Could you check a few things on this drawing? It's one solid part, dimensions in mm from its lowest x, y, z. A direction names the side the tool comes from. Round coordinates to 2 decimals unless told otherwise and drop trailing zeros. Loops run counter-clockwise (first coordinate to the right, second up) from the corner with the lowest first, then second, coordinate; pieces in that order, holes last. Notation, with made-up numbers: (-4, 83) -> (38, 83) arc R14 ccw to (38, 95) -> close; hole circle Ø5 at (53, 79.25). An arc over 180 degrees is marked (long way). Write each question's results on one line, items separated by ' | '.
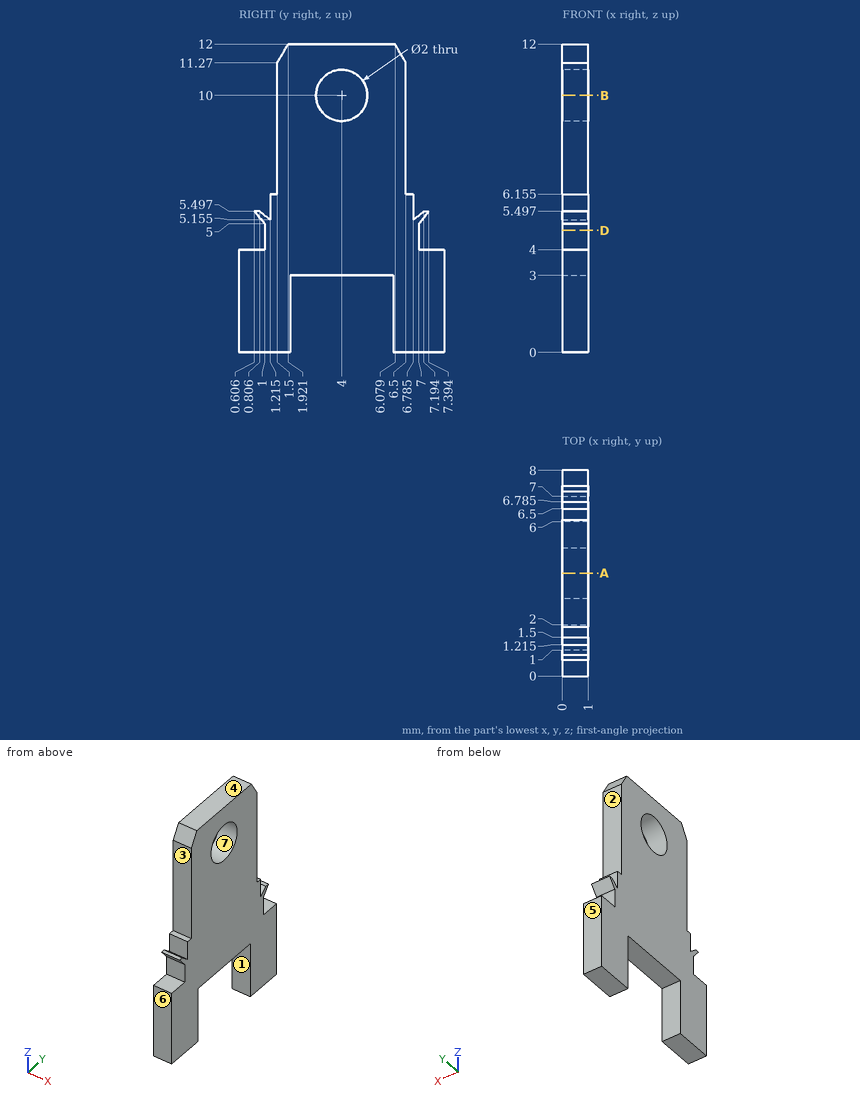
1) I want a section at B-B, the plane z = 10. Write out the boundary of the cut face in (x, y).
Model answer:
outline: (0, 1.5) -> (1, 1.5) -> (1, 3) -> (0, 3) -> close; (0, 5) -> (1, 5) -> (1, 6.5) -> (0, 6.5) -> close
2) For the marked faces 1, 2, 3 and 4, which set-ups out of +Z, -Z, +X, -X, +Y, -Y let a thin tool reach every point of the face, with its end or its side?
Model answer:
face 1: -Z, +X, -X | face 2: +Z, +X, -X, +Y | face 3: +Z, +X, -X, -Y | face 4: +Z, +X, -X, +Y, -Y
3) If we mould it in two halves opening along Y, with no side actions, what happens to the marked faces 5, 6 and 7? For each: released by +Y, released by -Y, zero draft, split by the parting line, or undercut.
Model answer:
face 5: released by +Y | face 6: released by -Y | face 7: undercut
4) I need wall thicknesses on line 1 (Z direction, x = 0.35, y = 4); line 2 (Y direction, x = 0.65, z = 10); line 3 (Y direction, x = 0.95, z = 2). Which ranges of each line are inside material? Lowest first, please.
Model answer:
line 1: z = 3 to 9, 11 to 12 | line 2: y = 1.5 to 3, 5 to 6.5 | line 3: y = 0 to 2, 6 to 8
5) I want a section at D-D, the plane z = 4.75. Write out the boundary of the cut face in (x, y).
Model answer:
outline: (0, 1) -> (1, 1) -> (1, 7) -> (0, 7) -> close
6) I want a section at A-A, the plane y = 4. Write out the boundary of the cut face in (x, z).
Model answer:
outline: (0, 3) -> (1, 3) -> (1, 9) -> (0, 9) -> close; (0, 11) -> (1, 11) -> (1, 12) -> (0, 12) -> close
7) I'm going to push flat-ended pins straight in: pin 1 (1.2 mm diameter, centred on y = 4, z = 10, fed in from +X); pin 2 (0.5 mm diameter, centred on x = 0.5, z = 6, fed in from +Y) (1 decimal); pin 3 (0.5 mm diameter, centred on x = 0.5, z = 5.5, fed in from -Y); pin 4 (0.5 mm diameter, centred on x = 0.5, y = 4, fed in from -Z). Where does each tip first touch, or does it pass through?
Model answer:
pin 1: passes through | pin 2: stops at y = 6.8 | pin 3: stops at y = 0.61 | pin 4: stops at z = 3
